```python
from build123d import *

# Parameters (mm, degrees)
SKETCH2_R           = 10
BOSS_EXTRUDE1_DEPTH = 1
SKETCH4_W           = 50
SKETCH4_H           = 24
BOSS_EXTRUDE2_DEPTH = 20


with BuildPart() as part:
    # Sketch2 → Boss-Extrude1 (new body)
    with BuildSketch(Plane(origin=(0, 0, 0), x_dir=(1, 0, 0), z_dir=(0, 1, 0))):
        with Locations(Location((0, 0, 0), (0, 0, 270))):
            Circle(SKETCH2_R)
    extrude(amount=-BOSS_EXTRUDE1_DEPTH)

    # Sketch4 → Boss-Extrude2 (add)
    with BuildSketch(Plane(origin=(0, -1, 0), x_dir=(1, 0, 0), z_dir=(0, 1, 0))):
        with Locations((-13, 0)):
            Rectangle(SKETCH4_W, SKETCH4_H)
    extrude(amount=-BOSS_EXTRUDE2_DEPTH)


solid = part.part
```
Geometry: final body of the model. Coordinates: model frame, mm. A direction names the side the tool comes from. Round coordinates to 2 decimals unless told otherwise and drop trailing zeros. Write each loop counter-clockwise with the first axis right and the second up, starting at its lowest first coordinate (ties: lowest second). Pieces come first, ordered by that corner, then holes.
Item 1: Material intervals for L1, parallel to Y at x = -33.5, z = 1, sorted ascending.
Item 2: Section query B-B (x = -35). Return loops of the section in (y, z), plus the area to 3 significant figures.
Item 3: Pin query (flat end, axial travel): P1, Ø6, axis at x = -31, z = -1, coming from the +Y side. Return the tip coordinate at first contact, or that it passes through.
Item 4: Section query D-D (z = 10.5). Return loops of the section in (x, y), plus the area to 3 significant figures.
Item 5: Section query C-C (z = 0). Return loops of the section in (x, y).
Item 6: Section query A-A (z = -6). Return loops of the section in (x, y), plus the area to 3 significant figures.
Item 7: Set-up query: faces 1 (the face through (-9.76, -0.49, -2.17)), 2 (the face through (-13, -11, 12)). Return all of +Z, -Z, +X, -X, +Y, -Y with unobstructed straight access to the full face (end or side cutting, diameter ignored); none if empty.
Completed:
1. L1: y = -21 to -1
2. outline: (-21, -12) - (-1, -12) - (-1, 12) - (-21, 12) - close
2. area: 480 mm2
3. P1: stops at y = -1
4. outline: (-38, -21) - (12, -21) - (12, -1) - (-38, -1) - close
4. area: 1,000 mm2
5. outline: (-38, -21) - (12, -21) - (12, -1) - (10, -1) - (10, 0) - (-10, 0) - (-10, -1) - (-38, -1) - close
6. outline: (-38, -21) - (12, -21) - (12, -1) - (8, -1) - (8, 0) - (-8, 0) - (-8, -1) - (-38, -1) - close
6. area: 1,020 mm2
7. face 1: +Y
7. face 2: +Z, +X, -X, +Y, -Y
